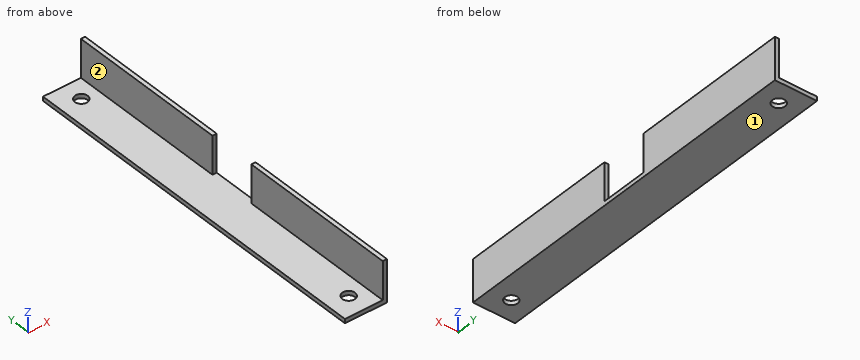
Solid Edge part; units mm, degrees
sketch "Sketch1" plane through (0, 0, 0) normal (0, -1, 0) x (1, 0, 0)
  line L0 (-36, 0) -> (0, 0)
  line L1 (0, 0) -> (0, 36)
  line L2 (0, 36) -> (4, 36)
  line L3 (4, 36) -> (4, -4)
  line L4 (4, -4) -> (-36, -4)
  line L5 (-36, -4) -> (-36, 0)
extrude "Protrusion1" add sketch "Sketch1" along normal mid plane 350
mirror "Mirror1" [suppressed]
sketch "Sketch2" plane through (-18, 0, 0) normal (0, 0, 1) x (0, -1, 0)
  circle A0 centre (-155, 2) radius 6.0641
  dimension "D1" = 155
  dimension "D2" = 155
extrude "Cutout1" cut sketch "Sketch2" against normal through all
mirror "Mirror2" about plane through (0, 0, 0) normal (0, -1, 0) of "Cutout1"
sketch "Sketch3" plane through (0, 0, 18) normal (-1, 0, 0) x (0, -1, 0)
  line L0 (-22.5, -18) -> (22.5, -18)
  line L1 (22.5, -18) -> (22.5, 18)
  line L2 (22.5, 18) -> (-22.5, 18)
  line L3 (-22.5, 18) -> (-22.5, -18)
  dimension "D1" = 22.5
extrude "Cutout2" cut sketch "Sketch3" against normal through all
properties material "Aluminium, 7075-T6"
Check sheet for the modelled part. Datum: model origin and axes. Units: mm. Face numbers are marked on the shaded views. A direction names the side the tool comes from. Give positions to 0.01 mm unless a question says otherwise; leave off trailing zeros. Write each loop counter-clockwise with the first axis right and the second up, starting at its lowest first coordinate (ties: lowest second). Pieces come first, ordered by that corner, then holes. Notation, with made-up numbers: (67, -34) -> (98, -34) arc R14 ccw to (98, -18) -> close; hole circle Ø10 at (68.25, -21.5). An arc over 180 degrees is marked (long way). Use CSV: the item, a comma, the result in double quotes. Start each with the question number.
Q1. Cross-section at C-C on x = -16. Enter the section's corners in (y, z).
Q2. Cross-section at B-B on z = 26. Enter the section's corners in (x, y).
Q3. Tool access check on the marked faces 1 and 2. Record the directions out of +Z, -Z, +X, -X, +Y, -Y that give a thin tool (end or side, any length) a straight path to the whole face; none if there is none.
Q4. Scan lines: line 1 along X through (y, z) = (-155, -1.65); line 2 along Y through (x, z) = (2.5, 1.5); line 3 along Z through (x, y) = (-0.5, -35.5). Record each from-to range of solid material in increasing order.
Q5. Depth check by flat-ended pin: P1, Ø11, axis at y = -75, z = 14, coming from the -X side; P2, Ø14, axis at x = -16, y = 155, coming from the +Z side; P3, Ø14, axis at x = -16, y = -155, coming from the -Z side. Enter the tip coordinate at first touch or a pass-through.
Q6. Cross-section at A-A on y = -155. Enter the section's corners in (x, z).
Working result:
1,outline,"(-175, -4) -> (-161.06, -4) -> (-161.06, 0) -> (-175, 0) -> close; (-148.94, -4) -> (148.94, -4) -> (148.94, 0) -> (-148.94, 0) -> close; (161.06, -4) -> (175, -4) -> (175, 0) -> (161.06, 0) -> close"
2,outline,"(0, -175) -> (4, -175) -> (4, -22.5) -> (0, -22.5) -> close; (0, 22.5) -> (4, 22.5) -> (4, 175) -> (0, 175) -> close"
3,face 1,"-Z, +X, -X, +Y, -Y"
3,face 2,"+Z, -X, +Y, -Y"
4,line 1,"x = -36 to -22.06, -9.94 to 4"
4,line 2,"y = -175 to -22.5, 22.5 to 175"
4,line 3,"z = -4 to 0"
5,P1,"stops at x = 0"
5,P2,"stops at z = 0"
5,P3,"stops at z = -4"
6,outline,"(-36, -4) -> (-22.06, -4) -> (-22.06, 0) -> (-36, 0) -> close; (-9.94, -4) -> (4, -4) -> (4, 36) -> (0, 36) -> (0, 0) -> (-9.94, 0) -> close"
